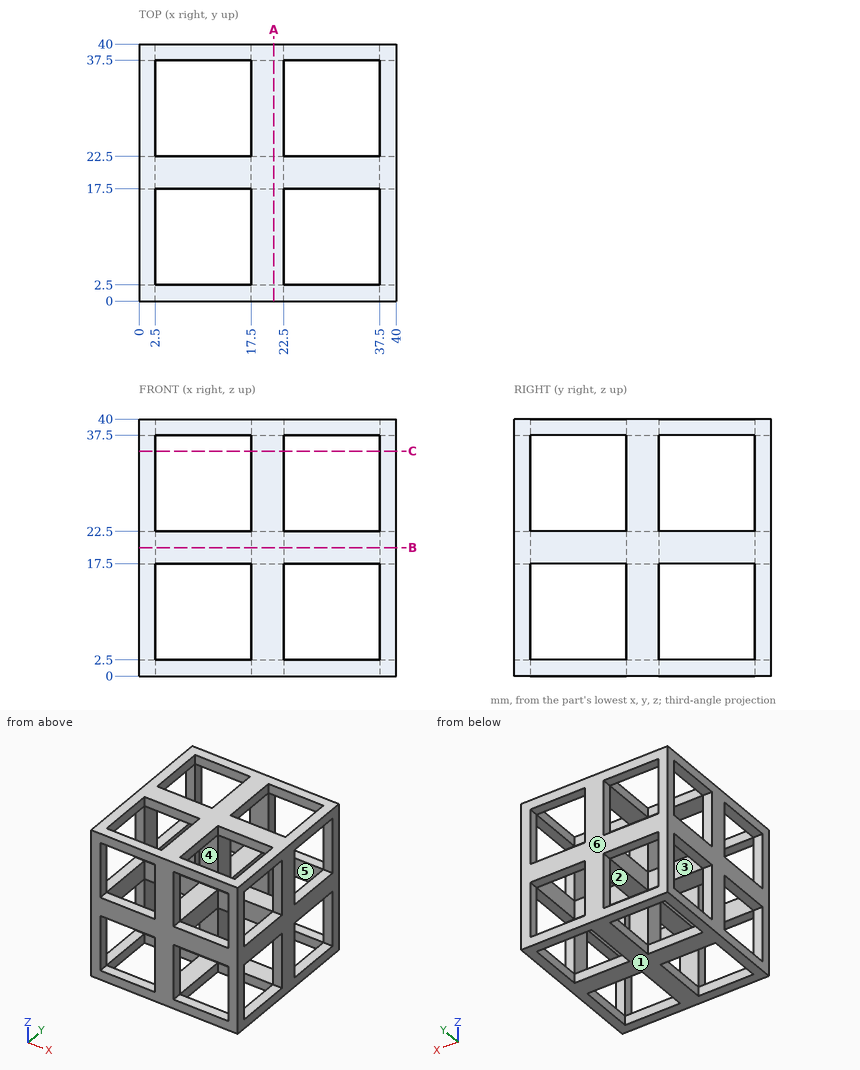
Check sheet for the drawn part. Datum: minimum x, y, z corner. Units: mm. A direction names the side the tool comes from. Round coordinates to 2 decimals unless told otherwise and drop trailing zeros. Write each loop counter-clockwise with the first axis right and the second up, starting at its lowest first coordinate (ties: lowest second). Pieces come first, ordered by that corner, then holes. Notation, with made-up numbers: (80.5, 44) - (93.5, 44) arc R20 ccw to (93.5, 54) - close; hole circle Ø5 at (-4.5, 40). An arc over 180 degrees is marked (long way). Return JSON: item names as keys, results as strings.
Q1. Cross-section at C-C (z = 35). Give the number of separate pieces and of enclosed holes in the cut face, then the cut area to 3 significant figures.
Returned:
{"separate pieces": "9", "enclosed holes": "0", "area": "100 mm²"}
Q2. Depth check by flat-ended pin: P1, Ø10, axis at x = 10, y = 28.5, coming from the +Z side; P2, Ø12, axis at x = 32, y = 11.5, coming from the -Z side. Enter the tip coordinate at first touch or a pass-through.
Returned:
{"P1": "passes through", "P2": "stops at z = 0"}
Q3. Cross-section at A-A (x = 21). Record the boundary of the cut face in (y, z), then the cut area to 3 significant figures.
Returned:
{"outline": "(0, 0) - (40, 0) - (40, 40) - (0, 40) - close; hole (2.5, 2.5) - (17.5, 2.5) - (17.5, 17.5) - (2.5, 17.5) - close; hole (2.5, 22.5) - (17.5, 22.5) - (17.5, 37.5) - (2.5, 37.5) - close; hole (22.5, 2.5) - (37.5, 2.5) - (37.5, 17.5) - (22.5, 17.5) - close; hole (22.5, 22.5) - (37.5, 22.5) - (37.5, 37.5) - (22.5, 37.5) - close", "area": "700 mm²"}
Q4. Scan line: L1, parallel to Z at x = 21, y = 16. Record every from-to range of solid material in increasing order. Write a range as from..to.
Returned:
{"L1": "z = 0..2.5, 17.5..22.5, 37.5..40"}
Q5. Draft check along Z on the marked faces 1, 2 and 3. Enter one of: released by +Z, released by -Z, zero draft, split by the parting line, or undercut.
Returned:
{"face 1": "released by -Z", "face 2": "undercut", "face 3": "zero draft"}
Q6. Access from +Z, -Z, +X, -X, +Y, -Y to the whole of each face (thin tool, end or side, straight path). Record for the marked faces 4, 5 and 6.
Returned:
{"face 4": "+X, -X", "face 5": "+Z, -Z", "face 6": "+Z, -Z, +X, -X, +Y"}
